```python
from build123d import *

# Parameters (mm, degrees)
SKETCH1_R                 = 1.6002
SKETCH1_R_2               = 11.0109
BOSS_EXTRUDE1_DEPTH       = 6.35
FILLET1_R                 = 2.54
F_6_32_TAPPED_HOLE1_D     = 2.7051
F_6_32_TAPPED_HOLE1_DEPTH = 9.38784
F_6_32_TAPPED_HOLE1_TIP   = 0.81269403
FILLET2_R                 = 1.5875


with BuildPart() as part:
    # Sketch1 → Boss-Extrude1 (new body)
    with BuildSketch(Plane.XY):
        with BuildLine():
            Line((0, 0), (35, 0))
            ThreePointArc((35, 0), (41.265093292, -18.936262305), (57.587844415, -30.399299417))
            ThreePointArc((57.587844415, -30.399299417), (60.74008766, -32.613036613), (61.95, -36.270000104))
            Line((61.95, -36.270000104), (17.5, -36.270000104))
            Line((17.5, -36.270000104), (17.5, -39.445000104))
            ThreePointArc((17.5, -39.445000104), (11.532534029, -62.925946747), (9.525, -87.070000104))
            Line((9.525, -87.070000104), (0, -87.070000104))
            Line((0, -87.070000104), (0, -36.270000104))
            Line((0, -36.270000104), (0, 0))
        make_face()
        with Locations((4.5, -4.5)):
            Circle(SKETCH1_R, mode=Mode.SUBTRACT)
        with Locations((17.5, -17.5)):
            Circle(SKETCH1_R_2, mode=Mode.SUBTRACT)
        with Locations((30.5, -30.5)):
            Circle(SKETCH1_R, mode=Mode.SUBTRACT)
    extrude(amount=BOSS_EXTRUDE1_DEPTH)

    # Fillet1
    fillet1_edges = [part.edges().sort_by_distance(p)[0] for p in [
        (0, 0, 3.175),
        (35, 0, 3.175),
        (9.525, -87.070000104, 3.175),
        (0, -87.070000104, 3.175),
    ]]
    fillet(fillet1_edges, radius=FILLET1_R)

    # #6-32 Tapped Hole1
    with Locations(Plane(origin=(0, -36.270000104, 0), x_dir=(-1, 0, 0), z_dir=(0, -1, 0))):
        with Locations((-22.58, -3.175), (-47.98, -3.175)):
            Hole(F_6_32_TAPPED_HOLE1_D / 2, depth=F_6_32_TAPPED_HOLE1_DEPTH)
            with Locations((0, 0, -(F_6_32_TAPPED_HOLE1_DEPTH + F_6_32_TAPPED_HOLE1_TIP / 2))):  # 118° drill point
                Cone(0, F_6_32_TAPPED_HOLE1_D / 2, F_6_32_TAPPED_HOLE1_TIP, mode=Mode.SUBTRACT)

    # Fillet2
    fillet2_edges = [part.edges().sort_by_distance(p)[0] for p in [
        (17.5, -36.270000104, 3.175),
    ]]
    fillet(fillet2_edges, radius=FILLET2_R)


solid = part.part
```
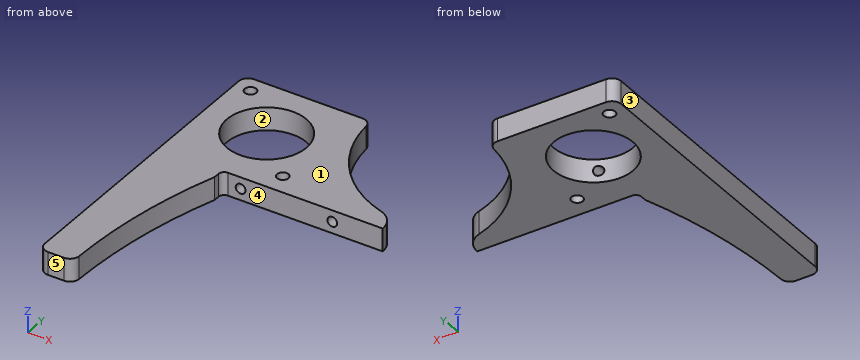
Part model, mm, in its own coordinate system. Face numbers are marked on the shaded views. A direction names the side the tool comes from. Coordinates: 2 decimals unless noted, no trailing zeros. Loops run counter-clockwise (first coordinate to the right, second up) from the corner with the lowest first, then second, coordinate; pieces in that order, holes last. Notation, with made-up numbers: (81, -24.5) - (134, -24.5) arc R34 cw to (134, 9.5) - close; hole circle Ø7 at (77, -4.5). An arc over 180 degrees is marked (long way). Write item = value, one per line. Start each with the question number.
Item 1: 3-axis set-ups, long thin cutter, end or side, ignore diameter. For the marked faces 4 and 5: which of +Z, -Z, +X, -X, +Y, -Y reach the whole face in a straight line?
Item 2: Cut at D-D, the plane x = 51. Give the cut face in (y, z), and give its area (3 significant figures).
Item 3: Cut at B-B, the plane y = -9.5. Give the cut face in (x, z).
Item 4: Mould opens along X. For the marked faces 1, 2 and 3 say: released by +X, released by -X, zero draft, split by the parting line, or undercut.
Item 5: Cut at C-C, the plane y = -75.5. Give the cut face in (x, z).
Item 6: Flat gauge pins, fed straight in: pin 1 Ø2 at (x, z) = (29.5, 3.5) entering from -Y; pin 2 Ø0.5 at (y, z) = (-38.5, 4.5) entering from +X; pin 3 Ø3 at (x, z) = (40, 3) entering from +Y. Where does each tip first touch, or does it go through?
Item 7: Cut at A-A, the plane x = 30.5. Give the cut face in (y, z), and give its area (3 significant figures).
Item 8: Wall check: L1, parallel to Y at x = 4.5, z = 4.5; L2, parallel to Y at x = 30.5, z = 1.75; L3, parallel to Z at x = 47.98, y = -29.5. Give the ranges that are in metal, low to high. Write a range as from..to.
The answers:
q1.face_4 = +Z, -Z, +X, -Y
q1.face_5 = +Z, -Z, +X, -X, -Y
q2.outline = (-36.27, 0) - (-27.57, 0) - (-27.57, 6.35) - (-36.27, 6.35) - close
q2.area = 55.3 mm2
q3.outline = (0, 0) - (9.93, 0) - (9.93, 6.35) - (0, 6.35) - close; (25.07, 0) - (36.45, 0) - (36.45, 6.35) - (25.07, 6.35) - close
q4.face_1 = zero draft
q4.face_2 = undercut
q4.face_3 = released by -X
q5.outline = (0, 0) - (9.98, 0) - (9.98, 6.35) - (0, 6.35) - close
q6.pin_1 = -36.27
q6.pin_2 = 17.5
q6.pin_3 = -14.49
q7.outline = (-36.27, 0) - (-32.1, 0) - (-32.1, 6.35) - (-36.27, 6.35) - close; (-28.9, 0) - (0, 0) - (0, 6.35) - (-28.9, 6.35) - close
q7.area = 210 mm2
q8.L1 = -87.07..-6.1, -2.9..0
q8.L2 = -36.27..-32.1, -28.9..0
q8.L3 = 0..1.82, 4.53..6.35
